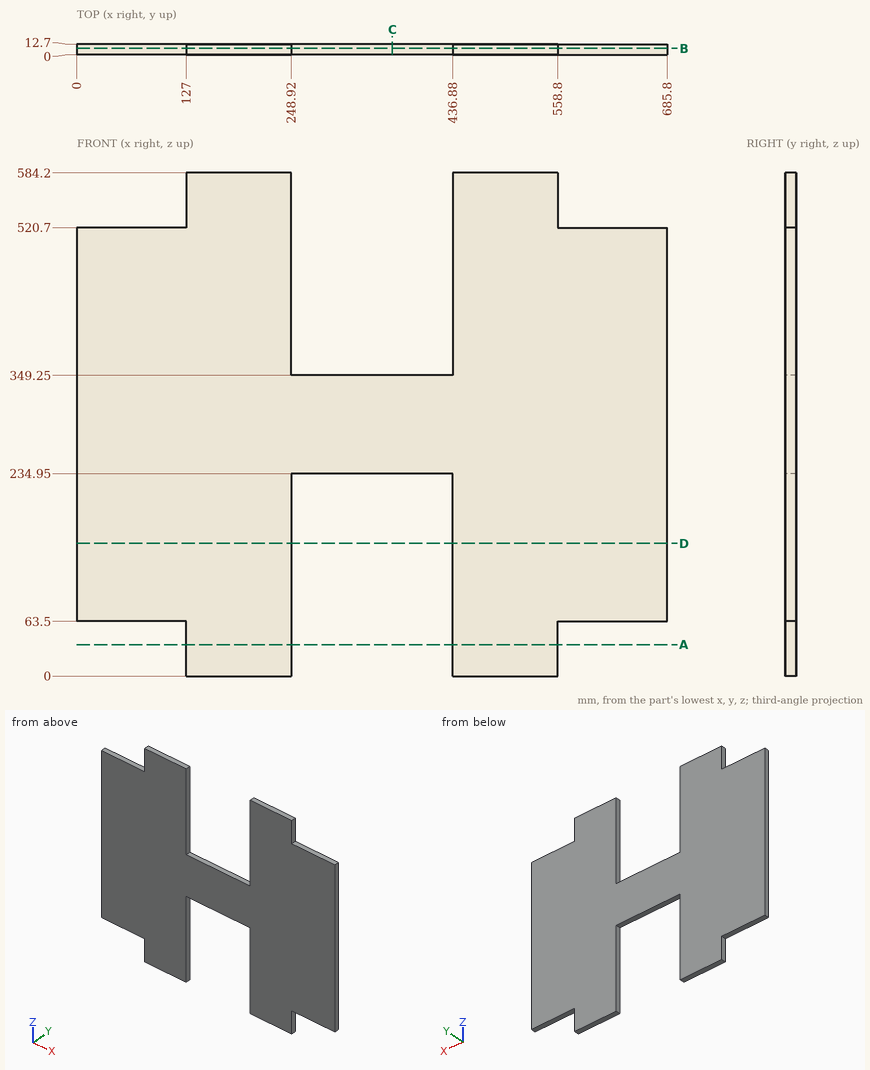
Here's the drawing with two shaded views (mm, measured from the low corner). I have some questions. Coordinates: 2 decimals unless noted, no trailing zeros. Order: outer loops, then holes, each group sorted by start corner. A loop starts at its lowest first (then second) coordinate and runs counter-clockwise, first axis right, second up. Notation, with made-up numbers: (16.5, 52.5) - (57.5, 52.5) arc R21 ccw to (57.5, 84.5) - close; hole circle Ø6 at (-1, 85). An arc over 180 degrees is marked (long way). Use CSV: the item, a comma, the result in double quotes. Start each with the question number.
1. Suppose I cut it at D-D on z = 154. List the corners of the cut face in (x, y) for me.
2. Please list where these lines run through material, in increasing order: line 1 (X direction, y = 6.5, z = 82.5); line 2 (Z direction, x = 296.5, y = 3.75); line 3 (Z direction, x = 85.5, y = 11). Write a range as from..to.
3. Suppose I cut it at A-A on z = 36.5. List the corners of the cut face in (x, y) for me, then the cut area to 3 significant figures.
4. Suppose I cut it at C-C on x = 366.5. List the corners of the cut face in (y, z) for me, then the cut area to 3 significant figures.
5. Suppose I cut it at B-B on y = 7.5. List the corners of the cut face in (x, z) for me.
6. I'm going to push flat-ended pins straight in: pin 1 (1.5 mm diameter, centred on x = 397.5, y = 10, fed in from +Z); pin 2 (6.5 mm diameter, centred on x = 626.5, y = 8, fed in from +Z); pin 3 (8 mm diameter, centred on x = 427, z = 246, fed in from -Y); pin 4 (4 mm diameter, centred on y = 5, z = 556.5, fed in from +X). Where does each tip first touch, or does it pass through?
Output:
1,outline,"(0, 0) - (248.92, 0) - (248.92, 12.7) - (0, 12.7) - close; (436.88, 0) - (685.8, 0) - (685.8, 12.7) - (436.88, 12.7) - close"
2,line 1,"x = 0..248.92, 436.88..685.8"
2,line 2,"z = 234.95..349.25"
2,line 3,"z = 63.5..520.7"
3,outline,"(127, 0) - (248.92, 0) - (248.92, 12.7) - (127, 12.7) - close; (436.88, 0) - (558.8, 0) - (558.8, 12.7) - (436.88, 12.7) - close"
3,area,"3,100 mm2"
4,outline,"(0, 234.95) - (12.7, 234.95) - (12.7, 349.25) - (0, 349.25) - close"
4,area,"1,450 mm2"
5,outline,"(0, 63.5) - (127, 63.5) - (127, 0) - (248.92, 0) - (248.92, 234.95) - (436.88, 234.95) - (436.88, 0) - (558.8, 0) - (558.8, 63.5) - (685.8, 63.5) - (685.8, 520.7) - (558.8, 520.7) - (558.8, 584.2) - (436.88, 584.2) - (436.88, 349.25) - (248.92, 349.25) - (248.92, 584.2) - (127, 584.2) - (127, 520.7) - (0, 520.7) - close"
6,pin 1,"stops at z = 349.25"
6,pin 2,"stops at z = 520.7"
6,pin 3,"stops at y = 0"
6,pin 4,"stops at x = 558.8"
